from build123d import *

# Parameters (mm, degrees)
SKETCH1_W                   = 152.4
SKETCH1_H                   = 127
BOSS_EXTRUDE1_DEPTH         = 3.175
SKETCH2_W                   = 69.85
SKETCH2_H                   = 9.525
BOSS_EXTRUDE2_DEPTH         = 38.1
BOSS_EXTRUDE3_DEPTH         = 101.6
BOSS_EXTRUDE4_START         = 101.6
SKETCH2_4_W                 = 69.85
SKETCH2_4_H                 = 9.525
SKETCH2_4_W_2               = 88.9
SKETCH2_4_H_2               = 88.9
BOSS_EXTRUDE4_DEPTH         = 12.7
CUT_EXTRUDE1_DEPTH          = 154.750010163
CUT_EXTRUDE1_DEPTH_BACK     = 5.08
SKETCH7_R                   = 17.9578
F_8_START                   = -50.8
F_8_CLEARANCE_SLOT1_2_DEPTH = 101.6
CIRPATTERN1_COUNT           = 4
FILLET2_R                   = 3.175
FILLET1_R                   = 12.7
CHAMFER1_SIZE               = 3.175
CHAMFER2_SIZE               = 9.525
CHAMFER4_SIZE               = 3.175
CHAMFER3_SIZE               = 0.79375
CHAMFER5_SIZE               = 0.79375
CHAMFER6_SIZE               = 0.396875


with BuildPart() as part:
    # Sketch1 → Boss-Extrude1 (new body)
    with BuildSketch(Plane(origin=(0, 0, 0), x_dir=(1, 0, 0), z_dir=(0, 1, 0))):
        Rectangle(SKETCH1_W, SKETCH1_H)
    extrude(amount=BOSS_EXTRUDE1_DEPTH)

    # Sketch2 → Boss-Extrude2 (add)
    with BuildSketch(Plane(origin=(0, 3.175, 0), x_dir=(1, 0, 0), z_dir=(0, 1, 0))):
        Polygon((-34.925, 53.975), (-53.975, 53.975), (-53.975, -53.975), (-34.925, -53.975), (-34.925, -44.45), (-44.45, -44.45), (-44.45, 44.45), (-34.925, 44.45), align=None)
        with Locations((0, 49.2125)):
            Rectangle(SKETCH2_W, SKETCH2_H)
        Polygon((53.975, 53.975), (34.925, 53.975), (34.925, 44.45), (44.45, 44.45), (44.45, -44.45), (34.925, -44.45), (34.925, -53.975), (53.975, -53.975), align=None)
        with Locations((0, -49.2125)):
            Rectangle(SKETCH2_W, SKETCH2_H)
    extrude(amount=BOSS_EXTRUDE2_DEPTH)

    # Sketch2<3> → Boss-Extrude3 (add)
    with BuildSketch(Plane(origin=(0, 3.175, 0), x_dir=(1, 0, 0), z_dir=(0, 1, 0))):
        Polygon((-34.925, 53.975), (-53.975, 53.975), (-53.975, -53.975), (-34.925, -53.975), (-34.925, -44.45), (-44.45, -44.45), (-44.45, 44.45), (-34.925, 44.45), align=None)
        Polygon((53.975, 53.975), (34.925, 53.975), (34.925, 44.45), (44.45, 44.45), (44.45, -44.45), (34.925, -44.45), (34.925, -53.975), (53.975, -53.975), align=None)
    extrude(amount=BOSS_EXTRUDE3_DEPTH)

    # Sketch2<4> → Boss-Extrude4 (add)
    with BuildSketch(Plane(origin=(0, 3.175, 0), x_dir=(1, 0, 0), z_dir=(0, 1, 0)).offset(BOSS_EXTRUDE4_START)):
        with Locations((0, 49.2125)):
            Rectangle(SKETCH2_4_W, SKETCH2_4_H)
        Polygon((-34.925, 53.975), (-53.975, 53.975), (-53.975, -53.975), (-34.925, -53.975), (-34.925, -44.45), (-44.45, -44.45), (-44.45, 44.45), (-34.925, 44.45), align=None)
        with Locations((0, -49.2125)):
            Rectangle(SKETCH2_4_W, SKETCH2_4_H)
        Polygon((53.975, 53.975), (34.925, 53.975), (34.925, 44.45), (44.45, 44.45), (44.45, -44.45), (34.925, -44.45), (34.925, -53.975), (53.975, -53.975), align=None)
        Rectangle(SKETCH2_4_W_2, SKETCH2_4_H_2)
    extrude(amount=BOSS_EXTRUDE4_DEPTH)

    # Sketch7 → Cut-Extrude1 (cut, two sides: drawn at the far end of the back side and taken through both)
    with BuildSketch(Plane(origin=(0, 117.475, 0), x_dir=(1, 0, 0), z_dir=(0, 1, 0)).offset(-CUT_EXTRUDE1_DEPTH_BACK)):
        with Locations(Location((0, 0, 0), (0, 0, 90))):
            Circle(SKETCH7_R)
    extrude(amount=CUT_EXTRUDE1_DEPTH + CUT_EXTRUDE1_DEPTH_BACK, mode=Mode.SUBTRACT)

    # #8 Clearance Slot1: read off the stored shape, not the designer's step
    # #8 Clearance Slot1 outline → #8 Clearance Slot1 (revolve, cut)
    with BuildSketch(Plane(origin=(66.675, 0, -50.8), x_dir=(1, 0, 0), z_dir=(0, 0, 1))):
        Polygon((0, 0), (2.8829, 0), (2.2479, 0.635), (2.2479, 2.54), (2.8829, 3.175), (0, 3.175), align=None)
    revolve(axis=Axis((66.675, 0, -50.8), (0, 1, 0)), mode=Mode.SUBTRACT)

    # 8 Clearance Slot1 2 outline → 8 Clearance Slot1 2 (cut)
    with BuildSketch(Plane.XY.offset(F_8_START)):
        Polygon((69.5579, 3.175), (63.7921, 3.175), (64.4271, 2.54), (64.4271, 0.635), (63.7921, 0), (69.5579, 0), (68.9229, 0.635), (68.9229, 2.54), align=None)
        Polygon((-64.4271, 2.54), (-63.7921, 3.175), (-69.5579, 3.175), (-68.9229, 2.54), (-68.9229, 0.635), (-69.5579, 0), (-63.7921, 0), (-64.4271, 0.635), align=None)
    extrude(amount=F_8_CLEARANCE_SLOT1_2_DEPTH, mode=Mode.SUBTRACT)

    # 8 Clearance Slot1 3 outline → 8 Clearance Slot1 3 (revolve, cut)
    with BuildSketch(Plane(origin=(66.675, 0, 50.8), x_dir=(1, 0, 0), z_dir=(0, 0, 1))):
        Polygon((0, 0), (2.8829, 0), (2.2479, 0.635), (2.2479, 2.54), (2.8829, 3.175), (0, 3.175), align=None)
    revolve(axis=Axis((66.675, 0, 50.8), (0, 1, 0)), mode=Mode.SUBTRACT)

    # 8 Clearance Slot1 4 outline → 8 Clearance Slot1 4 (revolve, cut)
    with BuildSketch(Plane(origin=(-66.675, 0, -50.8), x_dir=(1, 0, 0), z_dir=(0, 0, 1))):
        Polygon((0, 0), (2.8829, 0), (2.2479, 0.635), (2.2479, 2.54), (2.8829, 3.175), (0, 3.175), align=None)
    revolve(axis=Axis((-66.675, 0, -50.8), (0, 1, 0)), mode=Mode.SUBTRACT)

    # 8 Clearance Slot1 5 outline → 8 Clearance Slot1 5 (revolve, cut)
    with BuildSketch(Plane(origin=(-66.675, 0, 50.8), x_dir=(1, 0, 0), z_dir=(0, 0, 1))):
        Polygon((0, 0), (2.8829, 0), (2.2479, 0.635), (2.2479, 2.54), (2.8829, 3.175), (0, 3.175), align=None)
    revolve(axis=Axis((-66.675, 0, 50.8), (0, 1, 0)), mode=Mode.SUBTRACT)

    # Sketch11 → 1/2 (0.5) Diameter Hole1 (revolve, cut)
    with BuildSketch(Plane(origin=(25, 0, 0), x_dir=(0, 0, -1), z_dir=(1, 0, 0))):
        Polygon((0, 0), (0, 3.175), (6.985, 3.175), (6.35, 2.54), (6.35, 0.635), (6.985, 0), align=None)
    f_1_2_0_5_diameter_hole1 = revolve(axis=Axis((25, -6.35, 0), (0, 1, 0)), mode=Mode.SUBTRACT)

    # Sketch13 → #8 Clearance Hole2 (revolve, cut)
    with BuildSketch(Plane(origin=(25, 104.775, 0), x_dir=(0, 0, -1), z_dir=(1, 0, 0))):
        Polygon((0, 0), (0, 12.7), (2.5019, 12.7), (2.2479, 12.446), (2.2479, 0.635), (2.8829, 0), align=None)
    f_8_clearance_hole2 = revolve(axis=Axis((25, 98.425, 0), (0, 1, 0)), mode=Mode.SUBTRACT)

    # CirPattern1: 1/2 (0.5) Diameter Hole1, #8 Clearance Hole2 ×4 about axis
    cirpattern1_axis = Axis((0, 0, 0), (0, 1, 0))
    add([f_1_2_0_5_diameter_hole1.rotate(cirpattern1_axis, i * 360 / CIRPATTERN1_COUNT) for i in range(1, CIRPATTERN1_COUNT)], mode=Mode.SUBTRACT)
    add([f_8_clearance_hole2.rotate(cirpattern1_axis, i * 360 / CIRPATTERN1_COUNT) for i in range(1, CIRPATTERN1_COUNT)], mode=Mode.SUBTRACT)

    # Fillet2
    fillet2_edges = [part.edges().sort_by_distance(p)[0] for p in [
        (-44.45, 53.975, -44.45),
        (44.45, 53.975, -44.45),
        (44.45, 53.975, 44.45),
        (-44.45, 53.975, 44.45),
    ]]
    fillet(fillet2_edges, radius=FILLET2_R)

    # Fillet1
    fillet1_edges = [part.edges().sort_by_distance(p)[0] for p in [
        (53.975, 60.325, 53.975),
        (53.975, 60.325, -53.975),
        (-53.975, 60.325, -53.975),
        (-53.975, 60.325, 53.975),
        (76.2, 1.5875, 63.5),
        (-76.2, 1.5875, 63.5),
        (-76.2, 1.5875, -63.5),
        (76.2, 1.5875, -63.5),
    ]]
    fillet(fillet1_edges, radius=FILLET1_R)

    # Chamfer1
    chamfer1_edges = [part.edges().sort_by_distance(p)[0] for p in [
        (0, 3.175, -44.45),
        (-44.45, 3.175, 0),
        (0, 3.175, 44.45),
        (44.45, 3.175, 0),
        (43.52006403, 3.175, 43.52006403),
        (-43.52006403, 3.175, 43.52006403),
        (43.52006403, 3.175, -43.52006403),
        (-43.52006403, 3.175, -43.52006403),
        (53.975, 3.175, 0),
        (0, 3.175, 53.975),
        (-53.975, 3.175, 0),
        (0, 3.175, -53.975),
        (-50.255256121, 3.175, -50.255256121),
        (50.255256121, 3.175, -50.255256121),
        (50.255256121, 3.175, 50.255256121),
        (-50.255256121, 3.175, 50.255256121),
    ]]
    chamfer(chamfer1_edges, length=CHAMFER1_SIZE)

    # Chamfer2
    chamfer2_edges = [part.edges().sort_by_distance(p)[0] for p in [
        (-53.975, 117.475, 0),
        (0, 117.475, -53.975),
        (0, 117.475, 53.975),
        (53.975, 117.475, 0),
        (-50.255256121, 117.475, 50.255256121),
        (50.255256121, 117.475, 50.255256121),
        (50.255256121, 117.475, -50.255256121),
        (-50.255256121, 117.475, -50.255256121),
    ]]
    chamfer(chamfer2_edges, length=CHAMFER2_SIZE)

    # Chamfer4
    chamfer4_edges = [part.edges().sort_by_distance(p)[0] for p in [
        (-38.1, 104.775, -44.45),
        (-44.45, 104.775, 0),
        (44.45, 104.775, 0),
        (-38.1, 104.775, 44.45),
        (43.52006403, 104.775, 43.52006403),
        (-43.52006403, 104.775, 43.52006403),
        (43.52006403, 104.775, -43.52006403),
        (-43.52006403, 104.775, -43.52006403),
        (-34.925, 41.275, 49.2125),
        (-34.925, 41.275, -49.2125),
        (-34.925, 104.775, -49.2125),
        (-34.925, 104.775, 49.2125),
        (34.925, 41.275, -49.2125),
        (34.925, 104.775, -49.2125),
        (38.1, 104.775, 44.45),
        (34.925, 41.275, 49.2125),
        (34.925, 104.775, 49.2125),
        (38.1, 104.775, -44.45),
    ]]
    chamfer(chamfer4_edges, length=CHAMFER4_SIZE)

    # Chamfer3
    chamfer3_edges = [part.edges().sort_by_distance(p)[0] for p in [
        (0, 0, -63.5),
        (0, 3.175, -63.5),
        (76.2, 0, 0),
        (0, 0, 63.5),
        (-76.2, 0, 0),
        (72.480256121, 0, 59.780256121),
        (-72.480256121, 0, 59.780256121),
        (-72.480256121, 0, -59.780256121),
        (72.480256121, 0, -59.780256121),
        (76.2, 3.175, 0),
        (-76.2, 3.175, 0),
        (0, 3.175, 63.5),
        (72.480256121, 3.175, 59.780256121),
        (-72.480256121, 3.175, 59.780256121),
        (-72.480256121, 3.175, -59.780256121),
        (72.480256121, 3.175, -59.780256121),
    ]]
    chamfer(chamfer3_edges, length=CHAMFER3_SIZE)

    # Chamfer5
    chamfer5_edges = [part.edges().sort_by_distance(p)[0] for p in [
        (0, 117.475, 17.9578),
    ]]
    chamfer(chamfer5_edges, length=CHAMFER5_SIZE)

    # Chamfer6
    chamfer6_edges = [part.edges().sort_by_distance(p)[0] for p in [
        (0, 112.395, 17.9578),
    ]]
    chamfer(chamfer6_edges, length=CHAMFER6_SIZE)


solid = part.part
Could you check a few things on this model? Use its own coordinates, in mm. A direction names the side the tool comes from. Give positions to 0.01 mm unless a question says otherwise; leave off trailing zeros. Order: outer loops, then holes, each group sorted by start corner. A loop starts at its lowest first (then second) coordinate and runs counter-clockwise, first axis right, second up. Notation, with made-up numbers: (87, 68.25) - (131, 68.25) arc R15 ccw to (131, 83.25) - close; hole circle Ø9 at (75, -26). An arc over 180 degrees is marked (long way). One line per question, with ' | ' between items. Start each with the question number.
Item 1: I want a section at C-C on x = 0. Give the number of separate pieces and of enclosed holes in the cut face, then the cut area to 3 significant figures.
Item 2: I want a section at A-A on y = 50.5. Write out the boundary of the cut face in (x, z) (3 decimals).
Item 3: I'm going to push flat-ended pins straight in: pin 1 Ø25 at (x, y) = (13, 32) entering from +Z (3 decimals); pin 2 Ø10 at (x, z) = (25, 0) entering from -Y (3 decimals); pin 3 Ø4 at (x, y) = (50.5, 75.5) entering from +Z. Where does each tip first touch, or does it pass through?
Item 4: For faces 1 (the cylindrical face through (23.1, 111.2, -1.2)), 2 (the flat face through (34.925, 73, -49)), which set-ups out of +Z, -Z, +X, -X, +Y, -Y let a thin tool reach every point of the face, with its end or its side?
Item 5: I need wall thicknesses on probe 1 along Y at (x, z) = (-4.5, -9.5) (3 decimals); probe 2 along Y at (x, z) = (-4, -38) (3 decimals); probe 3 along X at (y, z) = (13, 23) (3 decimals). Which ranges of each line are inside material? Lowest first, please. Write a range as [from, to].
Item 6: Thinking about a two-plate mould opening in X: for faces 3 (the flat face through (19, 117.475, -1)), 4 (the cylindrical face through (-50.16, 57.86, 50.35)), 5 (the flat face through (0, 41.275, 49)), 6 (the conical face through (71.915, 0.127, -59.402)), which applies, pulls with the +X half, pulls with the -X half, needs draft (parallel to the pull), parting line crosses it, or undercut?
Item 7: I want a section at B-B on y = 27. Write out the boundary of the cut face in (x, z) (3 decimals).
Verdict:
1) separate pieces: 6 | enclosed holes: 0 | area: 2,050 mm^2
2) outline: (-53.975, -41.275) arc R12.7 ccw to (-41.275, -53.975) - (-34.925, -53.975) - (-34.925, -44.45) - (-41.275, -44.45) arc R3.175 cw to (-44.45, -41.275) - (-44.45, 41.275) arc R3.175 cw to (-41.275, 44.45) - (-34.925, 44.45) - (-34.925, 53.975) - (-41.275, 53.975) arc R12.7 ccw to (-53.975, 41.275) - close; (34.925, -53.975) - (41.275, -53.975) arc R12.7 ccw to (53.975, -41.275) - (53.975, 41.275) arc R12.7 ccw to (41.275, 53.975) - (34.925, 53.975) - (34.925, 44.45) - (41.275, 44.45) arc R3.175 cw to (44.45, 41.275) - (44.45, -41.275) arc R3.175 cw to (41.275, -44.45) - (34.925, -44.45) - close
3) pin 1: z = 53.975 | pin 2: y = 104.775 | pin 3: z = 51.72
4) face 1: +Y, -Y | face 2: +Z, -Z
5) probe 1: [0, 3.175], [104.775, 112.395] | probe 2: [0, 3.175], [104.775, 117.475] | probe 3: [-53.975, -44.45], [44.45, 53.975]
6) face 3: needs draft | face 4: pulls with the -X half | face 5: undercut | face 6: pulls with the +X half
7) outline: (-53.975, -41.275) arc R12.7 ccw to (-41.275, -53.975) - (41.275, -53.975) arc R12.7 ccw to (53.975, -41.275) - (53.975, 41.275) arc R12.7 ccw to (41.275, 53.975) - (-41.275, 53.975) arc R12.7 ccw to (-53.975, 41.275) - close; hole (-44.45, -41.275) arc R3.175 ccw to (-41.275, -44.45) - (41.275, -44.45) arc R3.175 ccw to (44.45, -41.275) - (44.45, 41.275) arc R3.175 ccw to (41.275, 44.45) - (-41.275, 44.45) arc R3.175 ccw to (-44.45, 41.275) - close
